Part model, mm, in its own coordinate system. Face numbers are marked on the shaded views. A direction names the side the tool comes from. Coordinates: 2 decimals unless noted, no trailing zeros. Loops run counter-clockwise (first coordinate to the right, second up) from the corner with the lowest first, then second, coordinate; pieces in that order, holes last. Notation, with made-up numbers: (17, -5) - (55, -5) arc R20 cw to (55, -1) - close; hole circle Ø6 at (64, 41). An arc over 180 degrees is marked (long way). Use a Markdown table: item, result. Add a question column.
1. Wall check: probe 1 along X at (y, z) = (-58, 53); probe 2 along Z at (x, y) = (66.5, -103); probe 3 along X at (y, z) = (-130.5, 165). Give the ranges that are in metal, low to high. Write a range as [from, to].
2. Drop flat-ended pins along their axis: pin 1 (8 mm diameter, centred on x = 84, z = 32.5, fed in from -Y); pin 2 (12 mm diameter, centred on x = 80.5, y = -157, fed in from +Z); pin 3 (4 mm diameter, centred on x = 118, y = -93, fed in from -Z); pin 4 (10 mm diameter, centred on y = -110, z = 41, fed in from -X). Give the stop position or say it passes through.
3. Band-saw the part on B-B, the plane z = -9. Give the cut face in (x, y), plus the area to 3 significant figures.
4. Pull direction X, two halves, no side cores. Call the marked faces 4, 5, 6 and 7: pulls with the +X half, pulls with the -X half, needs draft (parallel to the pull), parting line crosses it, or undercut.
5. Band-saw the part on A-A, the plane x = 143.5. Give the cut face in (y, z).
6. 3-axis set-ups, long thin cutter, end or side, ignore diameter. For the marked faces 1, 2 and 3: which of +Z, -Z, +X, -X, +Y, -Y reach the whole face in a straight line?
7. Band-saw the part on D-D, the plane z = 149. Give the cut face in (x, y).
from build123d import *

# Parameters (mm, degrees)
F1_DEPTH = 254
F2_R     = 5.72172
F3_DEPTH = 25.4
F5_DEPTH = 152.4
F6_R     = 39.082199
F6_R_2   = 34.497025
F7_DEPTH = 144.272


with BuildPart() as f1:
    # F0 (on Front) → F1 (new body)
    with BuildSketch(Plane.XZ):
        with BuildLine():
            Line((-5.052177, -58.048494), (5.052177, -58.048494))
            Line((5.052177, -58.048494), (20.930452, -58.048494))
            Line((20.930452, -58.048494), (20.930452, -49.800038))
            Line((20.930452, -49.800038), (13.052177, -49.800038))
            ThreePointArc((13.052177, -49.800038), (7.395323, -47.456893), (5.052177, -41.800038))
            Line((5.052177, -41.800038), (5.052177, 41.800038))
            ThreePointArc((5.052177, 41.800038), (7.395323, 47.456893), (13.052177, 49.800038))
            Line((13.052177, 49.800038), (20.930452, 49.800038))
            Line((20.930452, 49.800038), (20.930452, 58.048494))
            Line((20.930452, 58.048494), (5.052177, 58.048494))
            Line((5.052177, 58.048494), (-5.052177, 58.048494))
            Line((-5.052177, 58.048494), (-20.930452, 58.048494))
            Line((-20.930452, 58.048494), (-20.930452, 49.800038))
            Line((-20.930452, 49.800038), (-13.052177, 49.800038))
            ThreePointArc((-13.052177, 49.800038), (-7.395323, 47.456893), (-5.052177, 41.800038))
            Line((-5.052177, 41.800038), (-5.052177, -41.800038))
            ThreePointArc((-5.052177, -41.800038), (-7.395323, -47.456893), (-13.052177, -49.800038))
            Line((-13.052177, -49.800038), (-20.930452, -49.800038))
            Line((-20.930452, -49.800038), (-20.930452, -58.048494))
            Line((-20.930452, -58.048494), (-5.052177, -58.048494))
        make_face()
    extrude(amount=F1_DEPTH)

    # F2 (on face) → F3 (cut)
    with BuildSketch(Plane.XY.offset(58.048494)):
        with Locations((12.7, -14.956662)):
            Circle(F2_R)
        with Locations((12.7, -58.136662)):
            Circle(F2_R)
        with Locations((12.7, -101.316662)):
            Circle(F2_R)
        with Locations((12.7, -144.496662)):
            Circle(F2_R)
        with Locations((12.7, -187.676662)):
            Circle(F2_R)
        with Locations((12.7, -230.856662)):
            Circle(F2_R)
        with Locations((-12.7, -230.856662)):
            Circle(F2_R)
        with Locations((-12.7, -187.676662)):
            Circle(F2_R)
        with Locations((-12.7, -144.496662)):
            Circle(F2_R)
        with Locations((-12.7, -101.316662)):
            Circle(F2_R)
        with Locations((-12.7, -58.136662)):
            Circle(F2_R)
        with Locations((-12.7, -14.956662)):
            Circle(F2_R)
    extrude(amount=-F3_DEPTH, mode=Mode.SUBTRACT)

    # F4 (on face) → F5 (join)
    with BuildSketch(Plane.YZ.offset(5.052177)):
        with BuildLine():
            Line((-59.313846, -12.7), (-59.313846, 12.7))
            ThreePointArc((-59.313846, 12.7), (-64.893462, 26.170384), (-78.363846, 31.75))
            Line((-78.363846, 31.75), (-179.963846, 31.75))
            ThreePointArc((-179.963846, 31.75), (-193.434231, 26.170384), (-199.013846, 12.7))
            Line((-199.013846, 12.7), (-199.013846, -12.7))
            ThreePointArc((-199.013846, -12.7), (-193.434231, -26.170384), (-179.963846, -31.75))
            Line((-179.963846, -31.75), (-78.363846, -31.75))
            ThreePointArc((-78.363846, -31.75), (-64.893462, -26.170384), (-59.313846, -12.7))
        make_face()
        with BuildLine():
            ThreePointArc((-65.663846, -12.7), (-69.38359, -21.680256), (-78.363846, -25.4))
            Line((-78.363846, -25.4), (-179.963846, -25.4))
            ThreePointArc((-179.963846, -25.4), (-188.944102, -21.680256), (-192.663846, -12.7))
            Line((-192.663846, -12.7), (-192.663846, 12.7))
            ThreePointArc((-192.663846, 12.7), (-188.944102, 21.680256), (-179.963846, 25.4))
            Line((-179.963846, 25.4), (-78.363846, 25.4))
            ThreePointArc((-78.363846, 25.4), (-69.38359, 21.680256), (-65.663846, 12.7))
            Line((-65.663846, 12.7), (-65.663846, -12.7))
        make_face(mode=Mode.SUBTRACT)
    extrude(amount=F5_DEPTH)

    # F6 (on face) → F7 (join)
    with BuildSketch(Plane.XY.offset(31.75)):
        with Locations((88.872177, -129.163846)):
            Circle(F6_R)
        with Locations((88.872177, -129.163846)):
            Circle(F6_R_2, mode=Mode.SUBTRACT)
    extrude(amount=F7_DEPTH)


solid = f1.part
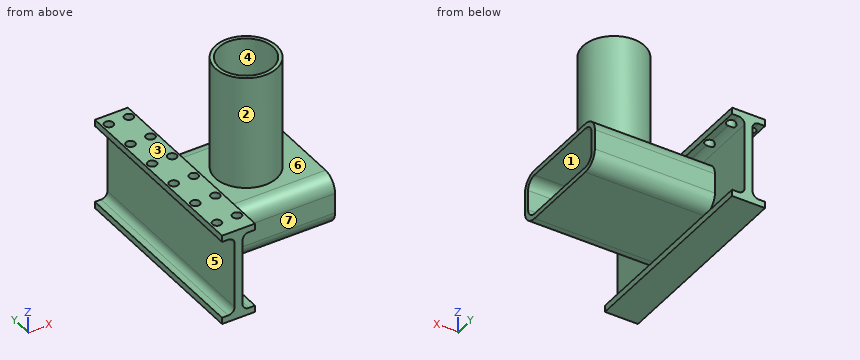
Geometry check:
| question | item | result |
|---|---|---|
| 1 | probe 1 | x = [-20.93, -18.42], [-6.98, 6.98], [18.42, 20.93] |
| 1 | probe 2 | z = [-31.75, -25.4], [25.4, 31.75] |
| 1 | probe 3 | x = [49.81, 54.4], [123.34, 127.93] |
| 2 | pin 1 | stops at y = -190.61 |
| 2 | pin 2 | stops at z = 176.02 |
| 2 | pin 3 | stops at z = -31.75 |
| 2 | pin 4 | stops at x = -6.24 |
| 3 | outline | (-5.05, -254) - (5.05, -254) - (5.05, -199.01) - (157.45, -199.01) - (157.45, -192.66) - (5.05, -192.66) - (5.05, -65.66) - (157.45, -65.66) - (157.45, -59.31) - (5.05, -59.31) - (5.05, 0) - (-5.05, 0) - close |
| 3 | area | 4,500 mm^2 |
| 4 | face 4 | undercut |
| 4 | face 5 | pulls with the -X half |
| 4 | face 6 | undercut |
| 4 | face 7 | needs draft |
| 5 | outline | (-199.01, -12.7) arc R19.05 ccw to (-179.96, -31.75) - (-78.36, -31.75) arc R19.05 ccw to (-59.31, -12.7) - (-59.31, 12.7) arc R19.05 ccw to (-78.36, 31.75) - (-179.96, 31.75) arc R19.05 ccw to (-199.01, 12.7) - close; hole (-192.66, -12.7) arc R12.7 ccw to (-179.96, -25.4) - (-78.36, -25.4) arc R12.7 ccw to (-65.66, -12.7) - (-65.66, 12.7) arc R12.7 ccw to (-78.36, 25.4) - (-179.96, 25.4) arc R12.7 ccw to (-192.66, 12.7) - close |
| 6 | face 1 | +X |
| 6 | face 2 | +Z |
| 6 | face 3 | +Z, -X, +Y, -Y |
| 7 | outline | circle Ø78.16 at (88.87, -129.16); hole circle Ø68.99 at (88.87, -129.16) |
